Input: dimensioned drawing with shaded views. Units: mm. Origin: part minimum x, y, z. A direction names the side the tool comes from. Round coordinates to 2 decimals unless told otherwise and drop trailing zeros. Loops run counter-clockwise (first coordinate to the right, second up) from the corner with the lowest first, then second, coordinate; pieces in that order, holes last. Notation, with made-up numbers: M -23.75,81 L 26.25,81 A28 ccw 26.25,112 Z; hole C -1,9 d8. An arc over 180 degrees is marked long. One line per item, written item: value.
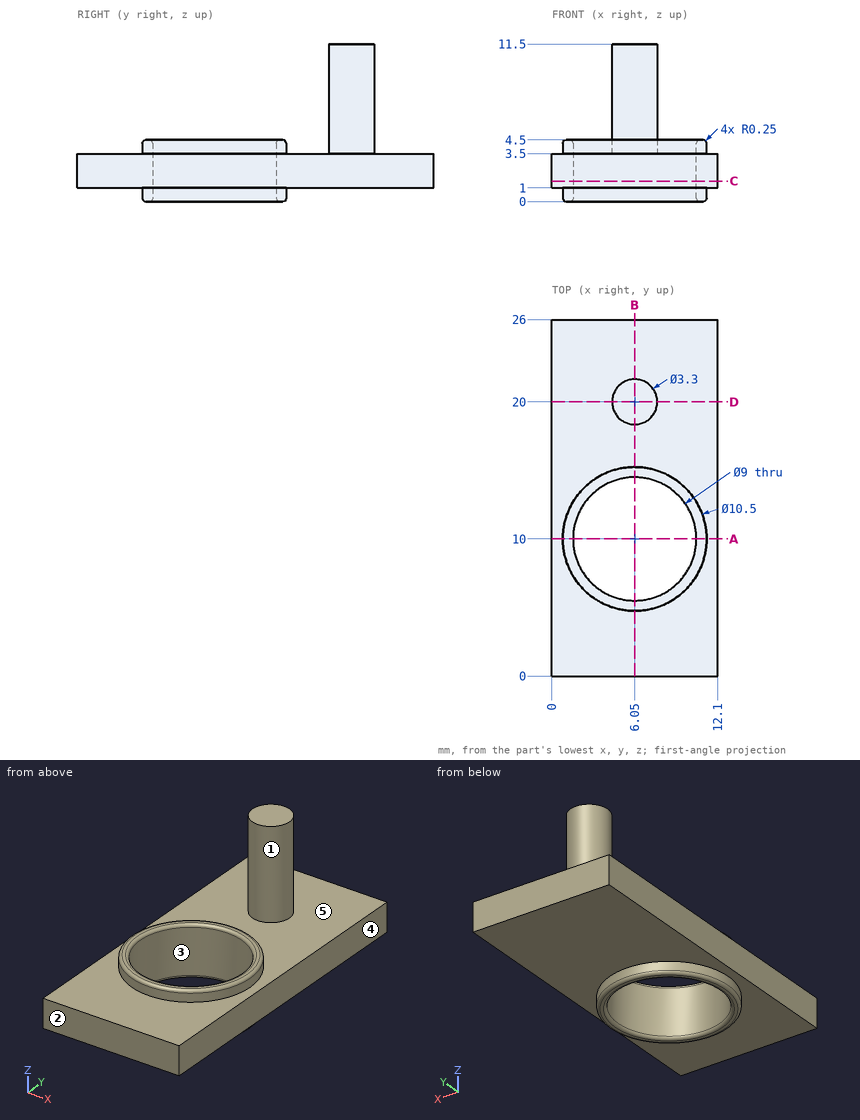
1. Section query B-B (x = 6.05). Return the cut outline in (y, z).
Report:
outline: M 0,1 L 4.75,1 L 4.75,0.25 A0.25 ccw 5,0 L 5.25,0 A0.25 ccw 5.5,0.25 L 5.5,4.25 A0.25 ccw 5.25,4.5 L 5,4.5 A0.25 ccw 4.75,4.25 L 4.75,3.5 L 0,3.5 Z; M 14.5,0.25 A0.25 ccw 14.75,0 L 15,0 A0.25 ccw 15.25,0.25 L 15.25,1 L 26,1 L 26,3.5 L 21.65,3.5 L 21.65,11.5 L 18.35,11.5 L 18.35,3.5 L 15.25,3.5 L 15.25,4.25 A0.25 ccw 15,4.5 L 14.75,4.5 A0.25 ccw 14.5,4.25 Z
2. Pin query (flat end, axial travel): pin 1 (1 mm diameter, centred on y = 17.5, z = 5.5, fed in from -X); pin 2 (4 mm diameter, centred on x = 7.5, y = 5, fed in from -Z); pin 3 (6 mm diameter, centred on x = 6, y = 15, fed in from +Z); pin 4 (4 mm diameter, centred on y = 21, z = 10, fed in from -X). Return the tip coordinate at first contact, or that it passes through.
Report:
pin 1: passes through
pin 2: stops at z = 0
pin 3: stops at z = 4.5
pin 4: stops at x = 4.4
3. Ray query, line 1 (Y direction, x = 6.05, z = 2.4); line 2 (Z direction, x = 9.5, y = 20.75); line 3 (Y direction, x = 9.75, z = 2). Return the intervals inside material, ascending. Write a range as [from, to].
Report:
line 1: y = [0, 5.5], [14.5, 26]
line 2: z = [1, 3.5]
line 3: y = [0, 7.44], [12.56, 26]
4. Section query C-C (z = 1.5). Return the cut outline in (x, y).
Report:
outline: M 0,0 L 12.1,0 L 12.1,26 L 0,26 Z; hole C 6.05,10 d9
5. Section query D-D (y = 20). Return the cut outline in (x, z).
Report:
outline: M 0,1 L 12.1,1 L 12.1,3.5 L 7.7,3.5 L 7.7,11.5 L 4.4,11.5 L 4.4,3.5 L 0,3.5 Z
6. Section query A-A (y = 10). Return the cut outline in (x, z).
Report:
outline: M 0,1 L 0.8,1 L 0.8,0.25 A0.25 ccw 1.05,0 L 1.3,0 A0.25 ccw 1.55,0.25 L 1.55,4.25 A0.25 ccw 1.3,4.5 L 1.05,4.5 A0.25 ccw 0.8,4.25 L 0.8,3.5 L 0,3.5 Z; M 10.55,0.25 A0.25 ccw 10.8,0 L 11.05,0 A0.25 ccw 11.3,0.25 L 11.3,1 L 12.1,1 L 12.1,3.5 L 11.3,3.5 L 11.3,4.25 A0.25 ccw 11.05,4.5 L 10.8,4.5 A0.25 ccw 10.55,4.25 Z
7. Pull-direction query (X, two-part tool) for the marked faces 3, 4 and 5; classes: released by +X, released by -X, zero draft, split by the parting line, or undercut.
Report:
face 3: undercut
face 4: released by +X
face 5: zero draft
8. Reachability of the marked faces 1 and 2 from +Z, -Z, +X, -X, +Y, -Y: full face, straight path, thin tool, end or side. Return the list, or none.
Report:
face 1: +Z
face 2: +Z, -Z, +X, -X, -Y
